from build123d import *

# Parameters (mm, degrees)
F1_DEPTH = 88
F2_R     = 5


with BuildPart() as f1:
    # F0 (on Top) → F1 (new body)
    with BuildSketch(Plane.XY):
        Polygon((-630, -15), (-630, -44), (630, -44), (630, -15), (660, -15), (660, 15), (630, 15), (630, 44), (-630, 44), (-630, 15), (-660, 15), (-660, -15), align=None)
    extrude(amount=F1_DEPTH)

    # F2
    f2_edges = [f1.edges().sort_by_distance(p)[0] for p in [
        (0, -44, 0),
        (0, -44, 88),
        (0, 44, 88),
        (630, -44, 44),
        (630, 44, 44),
        (0, 44, 0),
        (-630, 44, 44),
        (-630, -44, 44),
    ]]
    fillet(f2_edges, radius=F2_R)


solid = f1.part
CAD build for the part. Positions are in the model's coordinates, mm. A direction names the side the tool comes from. Coordinates: 2 decimals unless noted, no trailing zeros. Loops run counter-clockwise (first coordinate to the right, second up) from the corner with the lowest first, then second, coordinate; pieces in that order, holes last. Notation, with made-up numbers: (33.25, 32.5) - (66.25, 32.5) arc R21 cw to (66.25, 69.5) - close; hole circle Ø11 at (20.5, -8.5). An arc over 180 degrees is marked (long way). Use one line per item in the form item = value. Start each with the question number.
1) Tool access for faces 1 (the face through (645, -15, 43)), 2 (the face through (-645, 15, 43)), 3 (the face through (630, 27, 43)), 4 (the face through (9, 44, 43)), 5 (the face through (-645, -15, 43)): list every direction of +Z, -Z, +X, -X, +Y, -Y with a clear straight run to the whole face (end or side of a thin tool).
2) Band-saw the part on A-A (z = 57). Give the cut face in (x, y).
3) Flat gauge pins, fed straight in: pin 1 (7 mm diameter, centred on y = 30, z = 60.5, fed in from +X); pin 2 (7 mm diameter, centred on y = -26.5, z = 30.5, fed in from -X); pin 3 (15 mm diameter, centred on x = 639, z = 58, fed in from +Y). Where does each tip first touch, or does it go through?
4) Drill centre lines: L1, parallel to X at y = 18, z = 82; L2, parallel to Y at x = 449.5, z = 4. Where is each one in solid material? Low to high. Write a range as from..to.
Check values:
q1.face_1 = +Z, -Z, +X, -Y
q1.face_2 = +Z, -Z, -X, +Y
q1.face_3 = +Z, -Z, +X, +Y
q1.face_4 = +Z, -Z, +X, -X, +Y
q1.face_5 = +Z, -Z, -X, -Y
q2.outline = (-660, -15) - (-630, -15) - (-630, -39) arc R5 ccw to (-625, -44) - (625, -44) arc R5 ccw to (630, -39) - (630, -15) - (660, -15) - (660, 15) - (630, 15) - (630, 39) arc R5 ccw to (625, 44) - (-625, 44) arc R5 ccw to (-630, 39) - (-630, 15) - (-660, 15) - close
q3.pin_1 = 630
q3.pin_2 = -630
q3.pin_3 = 15
q4.L1 = -630..630
q4.L2 = -43.9..43.9
